The model under review builds one solid part; all positions refer to its coordinate system, in mm. Give positions to 0.01 mm unless a question says otherwise; leave off trailing zeros. Order: outer loops, then holes, each group sorted by start corner. A loop starts at its lowest first (then second) coordinate and runs counter-clockwise, first axis right, second up.
```python
from build123d import *

# Parameters (mm, degrees)
SKETCH2_W                                        = 155.575
SKETCH2_H                                        = 25.4
BOSS_EXTRUDE2_DEPTH                              = 4.7625
FILLET1_R                                        = 6.35
SKETCH3_R                                        = 1.5875
SKETCH3_R_2                                      = 2.38125
SKETCH3_R_3                                      = 3.175
SKETCH3_R_4                                      = 3.96875
SKETCH3_R_5                                      = 4.7625
CUT_EXTRUDE1_DEPTH                               = 158.706759624
CSK_FOR_M10_FLAT_HEAD_MACHINE_SCREW3_D           = 3.175
CSK_FOR_M10_FLAT_HEAD_MACHINE_SCREW3_CSINK_D     = 6.35
CSK_FOR_M10_FLAT_HEAD_MACHINE_SCREW3_CSINK_ANGLE = 90
CSK_FOR_M10_FLAT_HEAD_MACHINE_SCREW4_D           = 4.7625
CSK_FOR_M10_FLAT_HEAD_MACHINE_SCREW4_CSINK_D     = 7.9375
CSK_FOR_M10_FLAT_HEAD_MACHINE_SCREW4_CSINK_ANGLE = 90
CSK_FOR_M10_FLAT_HEAD_MACHINE_SCREW5_D           = 6.35
CSK_FOR_M10_FLAT_HEAD_MACHINE_SCREW5_CSINK_D     = 9.525
CSK_FOR_M10_FLAT_HEAD_MACHINE_SCREW5_CSINK_ANGLE = 90


with BuildPart() as part:
    # Sketch2 → Boss-Extrude2 (new body)
    with BuildSketch(Plane.XY):
        with Locations((77.7875, 12.7)):
            Rectangle(SKETCH2_W, SKETCH2_H)
    extrude(amount=BOSS_EXTRUDE2_DEPTH)

    # Fillet1
    fillet1_edges = [part.edges().sort_by_distance(p)[0] for p in [
        (0, 25.4, 2.38125),
        (155.575, 25.4, 2.38125),
        (155.575, 0, 2.38125),
        (0, 0, 2.38125),
    ]]
    fillet(fillet1_edges, radius=FILLET1_R)

    # Sketch3 → Cut-Extrude1 (cut, through all)
    with BuildSketch(Plane.XY.offset(4.7625)):
        with Locations((31.75, 12.7)):
            Circle(SKETCH3_R)
        with Locations((53.975, 12.7)):
            Circle(SKETCH3_R_2)
        with Locations((76.2, 12.7)):
            Circle(SKETCH3_R_3)
        with Locations((98.425, 12.7)):
            Circle(SKETCH3_R_4)
        with Locations((120.65, 12.7)):
            Circle(SKETCH3_R_5)
    extrude(amount=-CUT_EXTRUDE1_DEPTH, mode=Mode.SUBTRACT)

    # CSK for M10 Flat Head Machine Screw3 (through all)
    with Locations(Plane(origin=(31.75, 12.7, 4.7625), x_dir=(1, 0, 0), z_dir=(0, 0, 1))):
        with Locations((0, 0)):
            CounterSinkHole(CSK_FOR_M10_FLAT_HEAD_MACHINE_SCREW3_D / 2, CSK_FOR_M10_FLAT_HEAD_MACHINE_SCREW3_CSINK_D / 2, counter_sink_angle=CSK_FOR_M10_FLAT_HEAD_MACHINE_SCREW3_CSINK_ANGLE)

    # CSK for M10 Flat Head Machine Screw4 (through all)
    with Locations(Plane(origin=(53.975, 12.7, 4.7625), x_dir=(1, 0, 0), z_dir=(0, 0, 1))):
        with Locations((0, 0)):
            CounterSinkHole(CSK_FOR_M10_FLAT_HEAD_MACHINE_SCREW4_D / 2, CSK_FOR_M10_FLAT_HEAD_MACHINE_SCREW4_CSINK_D / 2, counter_sink_angle=CSK_FOR_M10_FLAT_HEAD_MACHINE_SCREW4_CSINK_ANGLE)

    # CSK for M10 Flat Head Machine Screw5 (through all)
    with Locations(Plane(origin=(76.2, 12.7, 4.7625), x_dir=(1, 0, 0), z_dir=(0, 0, 1))):
        with Locations((0, 0)):
            CounterSinkHole(CSK_FOR_M10_FLAT_HEAD_MACHINE_SCREW5_D / 2, CSK_FOR_M10_FLAT_HEAD_MACHINE_SCREW5_CSINK_D / 2, counter_sink_angle=CSK_FOR_M10_FLAT_HEAD_MACHINE_SCREW5_CSINK_ANGLE)

    # Sketch14 → CSK for M10 Flat Head Machine Screw6 (revolve, cut)
    with BuildSketch(Plane(origin=(98.425, 12.7, 4.7625), x_dir=(0, -1, 0), z_dir=(1, 0, 0))):
        Polygon((0, 0), (0, 4.7625), (3.96875, 4.7625), (3.96875, 1.5875), (5.55625, 0), align=None)
    revolve(axis=Axis((98.425, 12.7, 11.1125), (0, 0, -1)), mode=Mode.SUBTRACT)

    # Sketch15 → CSK for M10 Flat Head Machine Screw7 (revolve, cut)
    with BuildSketch(Plane(origin=(120.65, 12.7, 4.7625), x_dir=(0, -1, 0), z_dir=(1, 0, 0))):
        Polygon((0, 0), (0, 4.7625), (4.7625, 4.7625), (4.7625, 1.5875), (6.35, 0), align=None)
    revolve(axis=Axis((120.65, 12.7, 11.1125), (0, 0, -1)), mode=Mode.SUBTRACT)


solid = part.part
```
Item 1: Clearance check with flat-ended pins moving along their axes: pin 1 Ø8.5 at (x, y) = (120.65, 12.7) entering from +Z; pin 2 Ø9 at (x, y) = (98.425, 12.7) entering from +Z; pin 3 Ø1 at (y, z) = (22.5, 0.5) entering from +X. State where each tip first meets the part, or that it passes through.
Values found:
pin 1: passes through
pin 2: stops at z = 3.71
pin 3: stops at x = 154.85
Item 2: Take a section at D-D (x = 31.75). Give the boundary of the cut face in (y, z) (1 decimal).
Values found:
outline: (0, 0) - (11.1, 0) - (11.1, 3.2) - (9.5, 4.8) - (0, 4.8) - close; (14.3, 0) - (25.4, 0) - (25.4, 4.8) - (15.9, 4.8) - (14.3, 3.2) - close
Item 3: For line 1 (X direction, y = 12.7, z = 1.85) (1 decimal); line 2 (Y direction, x = 31.75, z = 1.2); line 3 (Y direction, x = 120.65, z = 1.8), list the stretches that pass through material, from the lowest coordinate up.
Values found:
line 1: x = 0 to 30.2, 33.3 to 51.6, 56.4 to 73, 79.4 to 94.5, 102.4 to 115.9, 125.4 to 155.6
line 2: y = 0 to 11.11, 14.29 to 25.4
line 3: y = 0 to 7.94, 17.46 to 25.4
Item 4: Draft analysis for pull direction Y (two halves, no side actions). For faces 1 (the cylindrical face through (1.81, 1.91, 2.41)), 2 (the cylindrical face through (153.764, 23.49, 2.415)), 3 (the cylindrical face through (95.276, 10.285, 1.61)), 4 (the conical face through (123.6, 16.6, 3.3)), state which applies: released by +Y, released by -Y, zero draft, split by the parting line, or undercut.
Values found:
face 1: released by -Y
face 2: released by +Y
face 3: undercut
face 4: undercut
Item 5: Take a section at B-B (z = 1.7). Give the number of separate pieces and of enclosed holes in the cut face, and give its area (3 significant figures).
Values found:
separate pieces: 1
enclosed holes: 5
area: 3,740 mm2
